Verification items for the finished model (mm, model axes). A direction names the side the tool comes from. Coordinates: 2 decimals unless noted, no trailing zeros. Write each loop counter-clockwise with the first axis right and the second up, starting at its lowest first coordinate (ties: lowest second). Pieces come first, ordered by that corner, then holes. Notation, with made-up numbers: (-14, -34) -> (1, -34) arc R15 cw to (1, -29) -> close; hole circle Ø11 at (30, 88). An arc over 180 degrees is marked (long way). Answer in a Markdown table with one row per item.
```python
from build123d import *

# Parameters (mm, degrees)
SKETCH_2_R                          = 79.5
SKETCH_3_R                          = 50
SKETCH_4_W                          = 60
SKETCH_4_H                          = 61.6
EXTRUDE_1_DEPTH                     = 31
EXTRUDE_2_DEPTH                     = 10
SKETCH_6_R                          = 6
EXTRUDE_3_DEPTH                     = 60
HOLE_WIZARD_3_8_0_375_1_D           = 9.525
HOLE_WIZARD_3_8_0_375_1_CSINK_D     = 10.795
HOLE_WIZARD_3_8_0_375_1_CSINK_ANGLE = 90
HOLE_WIZARD_1_4_0_25_1_D            = 6.35
HOLE_WIZARD_1_4_0_25_1_CSINK_D      = 7.62
HOLE_WIZARD_1_4_0_25_1_CSINK_ANGLE  = 90
HOLE_WIZARD_3_8_0_375_2_D           = 9.525
HOLE_WIZARD_3_8_0_375_2_CSINK_D     = 10.795
HOLE_WIZARD_3_8_0_375_2_CSINK_ANGLE = 90
HOLE_WIZARD_1_4_0_25_2_D            = 6.35
HOLE_WIZARD_1_4_0_25_2_CSINK_D      = 7.62
HOLE_WIZARD_1_4_0_25_2_CSINK_ANGLE  = 90


with BuildPart() as part:
    # 草图2 → 放样1 section 0
    with BuildSketch(Plane.XY):
        Circle(SKETCH_2_R)
    # 草图3 → 放样1 section 1
    with BuildSketch(Plane.XY.offset(23)):
        Circle(SKETCH_3_R)
    loft()

    # 草图4 → 凸台-拉伸1 (add)
    with BuildSketch(Plane.XY.offset(23)):
        Rectangle(SKETCH_4_W, SKETCH_4_H)
    extrude(amount=EXTRUDE_1_DEPTH)

    # 草图5 → 凸台-拉伸2 (add)
    with BuildSketch(Plane.ZY.offset(30)):
        with BuildLine():
            Line((23, 10), (43, 10))
            ThreePointArc((43, 10), (53, 0), (43, -10))
            Line((43, -10), (23, -10))
            Line((23, -10), (23, 10))
        make_face()
    extrude(amount=EXTRUDE_2_DEPTH)

    # 草图6 → 凸台-拉伸3 (add)
    with BuildSketch(Plane.ZY.offset(40)):
        with Locations((43, 0)):
            Circle(SKETCH_6_R)
    extrude(amount=EXTRUDE_3_DEPTH)

    # 3/8 (0.375) 直径孔1 (through all)
    with Locations(Plane.XY.offset(54)):
        with Locations((0, 0)):
            CounterSinkHole(HOLE_WIZARD_3_8_0_375_1_D / 2, HOLE_WIZARD_3_8_0_375_1_CSINK_D / 2, counter_sink_angle=HOLE_WIZARD_3_8_0_375_1_CSINK_ANGLE)

    # 1/4 (0.25) 直径孔1 (through all)
    with Locations(Plane.XY.offset(54)):
        with Locations((9, 9), (-9, 9), (-9, 0), (-9, -9), (9, -9), (9, 0)):
            CounterSinkHole(HOLE_WIZARD_1_4_0_25_1_D / 2, HOLE_WIZARD_1_4_0_25_1_CSINK_D / 2, counter_sink_angle=HOLE_WIZARD_1_4_0_25_1_CSINK_ANGLE)

    # 3/8 (0.375) 直径孔2 (through all)
    with Locations(Plane.XZ.offset(30.8)):
        with Locations((0, 39)):
            CounterSinkHole(HOLE_WIZARD_3_8_0_375_2_D / 2, HOLE_WIZARD_3_8_0_375_2_CSINK_D / 2, counter_sink_angle=HOLE_WIZARD_3_8_0_375_2_CSINK_ANGLE)

    # 1/4 (0.25) 直径孔2 (through all)
    with Locations(Plane(origin=(0, -30.8, 0), x_dir=(-1, 0, 0), z_dir=(0, -1, 0))):
        with Locations((9, -39), (-9, -39)):
            CounterSinkHole(HOLE_WIZARD_1_4_0_25_2_D / 2, HOLE_WIZARD_1_4_0_25_2_CSINK_D / 2, counter_sink_angle=HOLE_WIZARD_1_4_0_25_2_CSINK_ANGLE)


solid = part.part
```
1. Thickness scan on line 1 (Y direction, x = 9, z = 28) (3 decimals); line 2 (X direction, y = 23, z = 39) (1 decimal); line 3 (X direction, y = 0, z = 43.75) (1 decimal). Record the ranges inside material, lowest first. Write a range as from..to.
Geometry says:
| item | result |
|---|---|
| line 1 | -30.8..-12.175, -5.825..-3.175, 3.175..5.825, 12.175..30.8 |
| line 2 | -30..-12.2, -5.8..-4.8, 4.8..5.8, 12.2..30 |
| line 3 | -100..-12.2, -5.8..-4.8, 4.8..5.8, 12.2..30 |
2. Tool access check on faces 5 (the cylindrical face through (8.59, -19.43, 35.85)), 6 (the flat face through (-30, -14, 38)). Record the directions out of +Z, -Z, +X, -X, +Y, -Y that give a thin tool (end or side, any length) a straight path to the whole face; none if there is none.
Geometry says:
| item | result |
|---|---|
| face 5 | +Y, -Y |
| face 6 | +Z, -X |
3. Depth check by flat-ended pin: P1, Ø1, axis at x = -27.5, z = 42.5, coming from the -Y side; P2, Ø25, axis at y = -9, z = 42, coming from the +X side; P3, Ø3, axis at y = 31, z = 6.5, coming from the +X side. Enter the tip coordinate at first touch or a pass-through.
Geometry says:
| item | result |
|---|---|
| P1 | y = -30.8 |
| P2 | x = 30 |
| P3 | x = 66.3 |
4. Section check A-A, the plane x = 0. Record the boundary of the cut face in (y, z) (1 decimal).
Geometry says:
| item | result |
|---|---|
| outline | (-79.5, 0) -> (-4.8, 0) -> (-4.8, 34.2) -> (-30.2, 34.2) -> (-30.8, 33.6) -> (-30.8, 23) -> (-50, 23) -> close; (-30.8, 44.4) -> (-30.2, 43.8) -> (-4.8, 43.8) -> (-4.8, 53.4) -> (-5.4, 54) -> (-30.8, 54) -> close; (4.8, 0) -> (79.5, 0) -> (50, 23) -> (30.8, 23) -> (30.8, 34.2) -> (4.8, 34.2) -> close; (4.8, 43.8) -> (30.8, 43.8) -> (30.8, 54) -> (5.4, 54) -> (4.8, 53.4) -> close |
5. Mould release check, pull along Y, two halves, no side actions. Record for faces 1 (the flat face through (-35, 10, 33)), 2 (the cylindrical face through (-5.83, -8.86, 19.23)), 3 (the cylindrical face through (5.83, 4.56, 38.86)), 4 (the cylindrical face through (12.17, 0.14, 47.68)): released by +Y, released by -Y, zero draft, split by the parting line, or undercut.
Geometry says:
| item | result |
|---|---|
| face 1 | released by +Y |
| face 2 | undercut |
| face 3 | zero draft |
| face 4 | undercut |
6. Section check B-B, the plane z = 25. State how many separate pieces and enclosed holes the cut face has, plus the area to 3 significant figures.
Geometry says:
| item | result |
|---|---|
| separate pieces | 1 |
| enclosed holes | 7 |
| area | 3,630 mm^2 |
7. Section check D-D, the plane x = -86. Record the boundary of the cut face in (y, z).
Geometry says:
| item | result |
|---|---|
| outline | circle Ø12 at (0, 43) |
